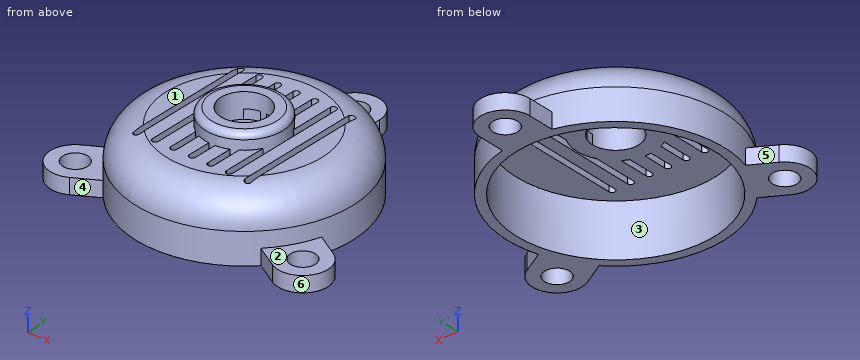
from build123d import *

# Parameters (mm, degrees)
SKETCH1_R           = 350
BOSS_EXTRUDE1_DEPTH = 200
SHELL4_T            = -30
BOSS_EXTRUDE2_START = -50
SKETCH2_R           = 40
BOSS_EXTRUDE2_DEPTH = 50
CIRPATTERN1_COUNT   = 3
FILLET1_R           = 100
CUT_EXTRUDE2_DEPTH  = 50
BOSS_EXTRUDE3_START = -30
SKETCH3_R           = 125
SKETCH3_R_2         = 75
BOSS_EXTRUDE3_DEPTH = 80
FILLET2_R           = 20
CUT_EXTRUDE1_START  = -50
SKETCH4_R           = 75
CUT_EXTRUDE1_DEPTH  = 50


with BuildPart() as part:
    # Sketch1 → Boss-Extrude1 (new body)
    with BuildSketch(Plane.XY):
        Circle(SKETCH1_R)
    extrude(amount=-BOSS_EXTRUDE1_DEPTH)

    # Shell4
    shell4_openings = [part.faces().sort_by_distance(p)[0] for p in [
        (0, 0, -200),
    ]]
    offset(amount=SHELL4_T, openings=shell4_openings, kind=Kind.INTERSECTION)

    # Sketch2 → Boss-Extrude2 (add)
    with BuildSketch(Plane(origin=(0, 0, -200), x_dir=(-1, 0, 0), z_dir=(0, 0, -1)).offset(BOSS_EXTRUDE2_START)):
        with BuildLine():
            ThreePointArc((80, 425), (0, 505), (-80, 425))
            Line((-80, 425), (-80, 340.734500748))
            ThreePointArc((-80, 340.734500748), (0, 350), (80, 340.734500748))
            Line((80, 340.734500748), (80, 425))
        make_face()
        with Locations((0, 425)):
            Circle(SKETCH2_R, mode=Mode.SUBTRACT)
    boss_extrude2 = extrude(amount=BOSS_EXTRUDE2_DEPTH)

    # CirPattern1: Boss-Extrude2 ×3 about axis
    cirpattern1_axis = Axis((0, 0, 0), (0, 0, 1))
    for i in range(1, CIRPATTERN1_COUNT):
        add(boss_extrude2.rotate(cirpattern1_axis, i * 360 / CIRPATTERN1_COUNT))

    # Fillet1
    fillet1_edges = [part.edges().sort_by_distance(p)[0] for p in [
        (-350, 0, 0),
    ]]
    fillet(fillet1_edges, radius=FILLET1_R)

    # Sketch5 → Cut-Extrude2 (cut)
    with BuildSketch(Plane.XY):
        with BuildLine():
            Line((-10, -200), (-10, 200))
            ThreePointArc((-10, 200), (0, 210), (10, 200))
            Line((10, 200), (10, -200))
            ThreePointArc((10, -200), (0, -210), (-10, -200))
        make_face()
        with BuildLine():
            Line((50, -200), (50, 200))
            ThreePointArc((50, 200), (60, 210), (70, 200))
            Line((70, 200), (70, -200))
            ThreePointArc((70, -200), (60, -210), (50, -200))
        make_face()
        with BuildLine():
            Line((110, -200), (110, 200))
            ThreePointArc((110, 200), (120, 210), (130, 200))
            Line((130, 200), (130, -200))
            ThreePointArc((130, -200), (120, -210), (110, -200))
        make_face()
        with BuildLine():
            Line((170, -200), (170, 200))
            ThreePointArc((170, 200), (180, 210), (190, 200))
            Line((190, 200), (190, -200))
            ThreePointArc((190, -200), (180, -210), (170, -200))
        make_face()
        with BuildLine():
            Line((-70, -200), (-70, 200))
            ThreePointArc((-70, 200), (-60, 210), (-50, 200))
            Line((-50, 200), (-50, -200))
            ThreePointArc((-50, -200), (-60, -210), (-70, -200))
        make_face()
        with BuildLine():
            Line((-130, -200), (-130, 200))
            ThreePointArc((-130, 200), (-120, 210), (-110, 200))
            Line((-110, 200), (-110, -200))
            ThreePointArc((-110, -200), (-120, -210), (-130, -200))
        make_face()
        with BuildLine():
            Line((-190, -200), (-190, 200))
            ThreePointArc((-190, 200), (-180, 210), (-170, 200))
            Line((-170, 200), (-170, -200))
            ThreePointArc((-170, -200), (-180, -210), (-190, -200))
        make_face()
    extrude(amount=-CUT_EXTRUDE2_DEPTH, mode=Mode.SUBTRACT)

    # Sketch3 → Boss-Extrude3 (add)
    with BuildSketch(Plane.XY.offset(BOSS_EXTRUDE3_START)):
        with Locations(Location((0, 0, 0), (0, 0, 151.642363424))):
            Circle(SKETCH3_R)
        with Locations(Location((0, 0, 0), (0, 0, 158.960530219))):
            Circle(SKETCH3_R_2, mode=Mode.SUBTRACT)
    extrude(amount=BOSS_EXTRUDE3_DEPTH)

    # Fillet2
    fillet2_edges = [part.edges().sort_by_distance(p)[0] for p in [
        (110, -59.371710435, 50),
    ]]
    fillet(fillet2_edges, radius=FILLET2_R)

    # Sketch4 → Cut-Extrude1 (cut)
    with BuildSketch(Plane.XY.offset(CUT_EXTRUDE1_START)):
        Circle(SKETCH4_R)
    extrude(amount=CUT_EXTRUDE1_DEPTH, mode=Mode.SUBTRACT)


solid = part.part
The listing builds one solid part. Answer for the finished solid, in the listing's coordinates (mm). Face numbers are marked on the shaded views. A direction names the side the tool comes from. Round coordinates to 2 decimals unless told otherwise and drop trailing zeros. Loops run counter-clockwise (first coordinate to the right, second up) from the corner with the lowest first, then second, coordinate; pieces in that order, holes last. Notation, with made-up numbers: M 65,59.5 L 122,59.5 A23 cw 122,91.5 Z; hole C -14.5,6 d10. An arc over 180 degrees is marked long. Return JSON: item names as keys, results as strings.
Q1. Which of the six approach directions +Z, -Z, +X, -X, +Y, -Y give full straight-line access (tool end or side, diameter ignored) to the marked faces 1, 2 and 3?
Results list:
{"face 1": "+Z, -X, +Y, -Y", "face 2": "+Z, +X, -Y", "face 3": "-Z"}
Q2. The mould has two halves that part along Y. Classify the marked faces 4, 5 and 6: released by +Y, released by -Y, zero draft, split by the parting line, or undercut.
Results list:
{"face 4": "released by -Y", "face 5": "undercut", "face 6": "split by the parting line"}
Q3. Find section A-A, the plane z = -58. Determine the outline of the cut face in (x, y), plus the area to 3 significant figures.
Results list:
{"outline": "C 0,0 d681.5; hole C 0,0 d640", "area": "43,100 mm2"}
Q4. Each of these flat-tipped pins is pushed along its axis until it touches: pin 1 Ø8 at (x, y) = (-163, -128.5) entering from -Z; pin 2 Ø18 at (x, y) = (-207.5, 44.5) entering from +Z; pin 3 Ø24 at (y, z) = (148, -12) entering from -X. Where does it stop, or does it pass through?
Results list:
{"pin 1": "stops at z = -30", "pin 2": "stops at z = 0", "pin 3": "stops at x = -279.24"}
Q5. Find the intervals of material crossed by line 1 along Y through (x, z) = (0, -177); line 2 along X through (y, z) = (0, 21); line 3 along Y through (x, z) = (-236.5, -107), in increasing order. Write a range as from..to.
Results list:
{"line 1": "y = -350..-320, 320..385, 465..505", "line 2": "x = -125..-75, 75..125", "line 3": "y = -258.01..-215.56, 215.56..258.01"}
